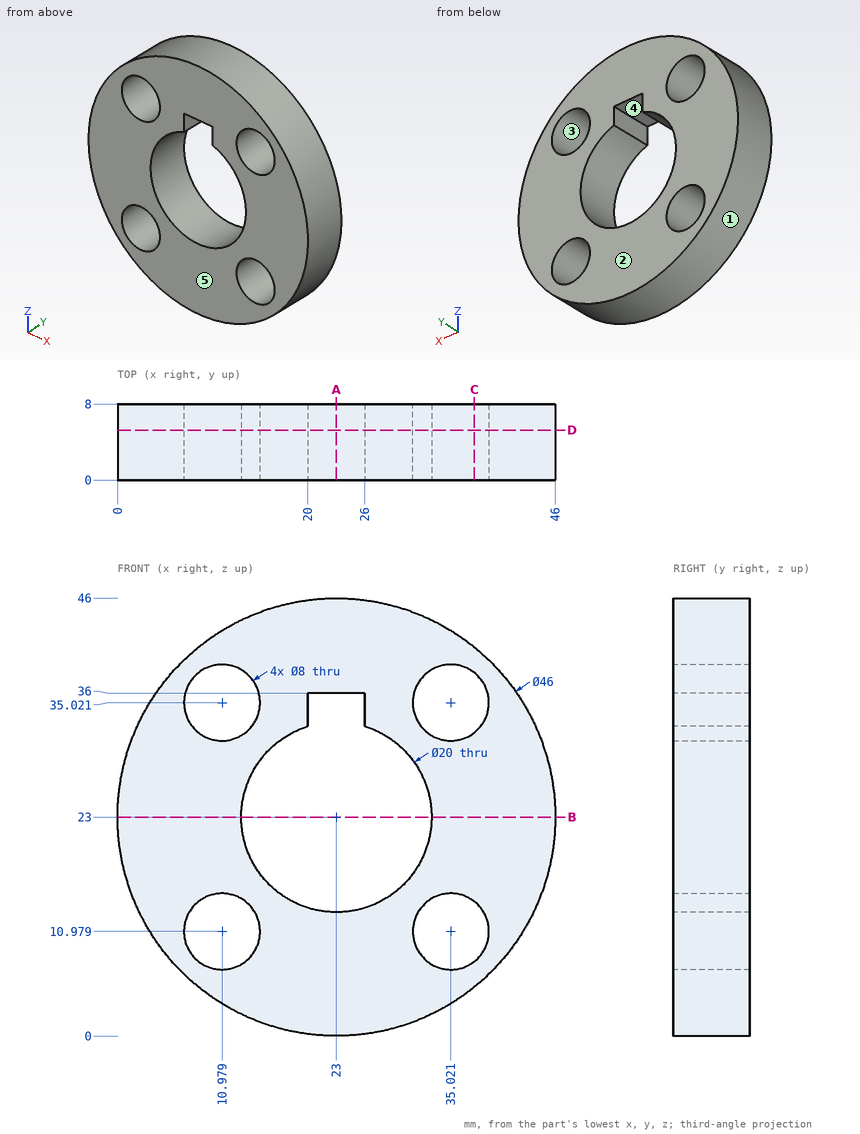
Study the drawing (mm; zero at the part's minimum x, y, z) and answer. A direction names the side the tool comes from. Round coordinates to 2 decimals unless told otherwise and drop trailing zeros. Loops run counter-clockwise (first coordinate to the right, second up) from the corner with the lowest first, then second, coordinate; pieces in that order, holes last. Notation, with made-up numbers: (80, -6) -> (137, -6) arc R20 cw to (137, -2) -> close; hole circle Ø8 at (15, 80.25). An arc over 180 degrees is marked (long way). One line per item, written item: value.
1) Consider L1, parallel to Z at x = 35.5, y = 2.25; L2, parallel to Z at x = 37.5, y = 7; L3, parallel to Z at x = 22.5, y = 6.5. Determine where each line is inside the solid, lowest interval first. Write a range as [from, to].
Answer list:
L1: z = [3.69, 7.01], [14.95, 31.05], [38.99, 42.31]
L2: z = [5.15, 7.84], [14.12, 31.88], [38.16, 40.85]
L3: z = [0.01, 13.01], [36, 45.99]
2) The mould has two halves that part along X. Classify the marked faces 1, 2 and 3: pulls with the +X half, pulls with the -X half, needs draft (parallel to the pull), parting line crosses it, or undercut.
Answer list:
face 1: parting line crosses it
face 2: needs draft
face 3: undercut
3) A cutting plane is placed at D-D (y = 5.25). Determine the outline of the cut face in (x, z).
Answer list:
outline: circle Ø46 at (23, 23); hole circle Ø8 at (10.98, 10.98); hole circle Ø8 at (10.98, 35.02); hole (20, 32.54) arc R10 ccw (long way) to (26, 32.54) -> (26, 36) -> (20, 36) -> close; hole circle Ø8 at (35.02, 10.98); hole circle Ø8 at (35.02, 35.02)
4) For the marked faces 4 and 5, determine the directions among +Z, -Z, +X, -X, +Y, -Y from which every point of the face is accessible in a straight line to the end or side of a thin tool.
Answer list:
face 4: +Y, -Y
face 5: +Z, -Z, +X, -X, -Y
5) A cutting plane is placed at B-B (z = 23). Determine the outline of the cut face in (x, y), and give its area (3 significant figures).
Answer list:
outline: (0, 0) -> (13, 0) -> (13, 8) -> (0, 8) -> close; (33, 0) -> (46, 0) -> (46, 8) -> (33, 8) -> close
area: 208 mm²
6) Flat-ended cylindrical pins translate along their axes: P1, Ø3, axis at y = 2.5, z = 40.5, coming from the +X side; P2, Ø7, axis at x = 10.98, z = 35.02, coming from the +Y side; P3, Ø3, axis at x = 24.5, y = 5, coming from the -Z side; P4, Ø1, axis at x = 28, y = 3.5, coming from the -Z side. Find the tip coordinate at first contact, or state that the pin passes through.
Answer list:
P1: stops at x = 39.52
P2: passes through
P3: stops at z = 0
P4: stops at z = 0.44
7) A cutting plane is placed at C-C (x = 37.5). Determine the outline of the cut face in (y, z).
Answer list:
outline: (0, 5.15) -> (8, 5.15) -> (8, 7.84) -> (0, 7.84) -> close; (0, 14.12) -> (8, 14.12) -> (8, 31.88) -> (0, 31.88) -> close; (0, 38.16) -> (8, 38.16) -> (8, 40.85) -> (0, 40.85) -> close
8) A cutting plane is placed at A-A (x = 23). Determine the outline of the cut face in (y, z).
Answer list:
outline: (0, 0) -> (8, 0) -> (8, 13) -> (0, 13) -> close; (0, 36) -> (8, 36) -> (8, 46) -> (0, 46) -> close
